Here's how the part is built. I have some questions about the finished solid (model axes, mm). Round coordinates to 2 decimals unless told otherwise and drop trailing zeros. Write each loop counter-clockwise with the first axis right and the second up, starting at its lowest first coordinate (ties: lowest second). Pieces come first, ordered by that corner, then holes. Notation, with made-up numbers: (44, 38) -> (60, 38) arc R24 ccw to (60, 53) -> close; hole circle Ø1 at (67, 41.5). An arc over 180 degrees is marked (long way). Answer in a Markdown table with one row per item.
Autodesk Inventor part; units mm, degrees
ref_plane "YZ Plane" through (0, 0, 0) normal (1, 0, 0) x (0, 1, 0)
ref_plane "XZ Plane" through (0, 0, 0) normal (0, 1, 0) x (-1, 0, 0)
ref_plane "XY Plane" through (0, 0, 0) normal (0, 0, 1) x (1, 0, 0)
sketch "Sketch1" plane through (0, 0, 0) normal (0, 1, 0) x (-1, 0, 0)
  line L0 (0, 0) -> (26.75, 0) construction
  line L1 (0, -9.75) -> (26.75, -9.75)
  line L2 (26.75, 9.75) -> (0, 9.75)
  arc A0 (0, 9.75) -> (0, -9.75) centre (0, 0) ccw
  arc A1 (26.75, -9.75) -> (26.75, 9.75) centre (26.75, 0) ccw
  point P0 (13.375, 0)
  dimension "d0" = 26.75
  dimension "d1" = 19.5
extrude "Extrusion1" add sketch "Sketch1" along normal blind 2 and the other way blind 1
sketch "Sketch2" plane through (0, 2, 0) normal (0, 1, 0) x (1, 0, 0)
  point P0 (0, 0)
hole "Hole1" at (0, 2, 0) direction (0, -1, 0) diameter 6.6 end up to surface
properties part number "SP36V1 Traba Cierre"
1) I need wall thicknesses on line 1 (Z direction, x = 0, y = 0.95); line 2 (X direction, y = -0.05, z = 0); line 3 (X direction, y = 0.85, z = -2.75). Which ranges of each line are inside material? Lowest first, please. Write a range as [from, to].
Response:
| item | result |
|---|---|
| line 1 | z = [-9.75, -3.3], [3.3, 9.75] |
| line 2 | x = [-36.5, -3.3], [3.3, 9.75] |
| line 3 | x = [-36.1, -1.82], [1.82, 9.35] |
2) We'd pull the mould along X, two halves only. Please class faces 1 (the face through (-36.498, 0.479, 0.214)), 2 (the face through (9.748, 0.479, -0.214)), 3 (the face through (-2.23, 0.48, -2.43)), 4 (the face through (-13, -1, 0)): +X half, -X half, draft (parallel to the pull), parting line (faces both ways), or undercut.
Response:
| item | result |
|---|---|
| face 1 | -X half |
| face 2 | +X half |
| face 3 | undercut |
| face 4 | draft |
3) I want a section at D-D, the plane z = -6. List the corners of the cut face in (x, y) for me.
Response:
| item | result |
|---|---|
| outline | (-34.44, -1) -> (7.69, -1) -> (7.69, 2) -> (-34.44, 2) -> close |
4) I want a section at C-C, the plane x = -30.5. List the corners of the cut face in (y, z) for me, and give its area (3 significant figures).
Response:
| item | result |
|---|---|
| outline | (-1, -9) -> (2, -9) -> (2, 9) -> (-1, 9) -> close |
| area | 54.0 mm^2 |
5) I want a section at B-B, the plane y = 0.55. List the corners of the cut face in (x, z) for me.
Response:
| item | result |
|---|---|
| outline | (-26.75, -9.75) -> (0, -9.75) arc R9.75 ccw to (0, 9.75) -> (-26.75, 9.75) arc R9.75 ccw to start; hole circle Ø6.6 at (0, 0) |
6) I want a section at A-A, the plane z = 0. List the corners of the cut face in (x, y) for me, and give its area (3 significant figures).
Response:
| item | result |
|---|---|
| outline | (-36.5, -1) -> (-3.3, -1) -> (-3.3, 2) -> (-36.5, 2) -> close; (3.3, -1) -> (9.75, -1) -> (9.75, 2) -> (3.3, 2) -> close |
| area | 119 mm^2 |
